Autodesk Inventor part; units mm, degrees
ref_plane "Work Plane1" through (-2, 0, -9) normal (-1, 0, 0) x (0, 0, 1)
ref_plane "Work Plane2" through (-2.4, 12.4824, -5.5) normal (0, 0, 1) x (1, 0, 0)
ref_plane "YZ Plane" through (0, 0, 0) normal (1, 0, 0) x (0, 1, 0)
sketch "Sketch1" plane through (0, 0, 0) normal (0, 1, 0) x (-1, 0, 0)
  line L0 (0, 0) -> (4, 0)
  line L1 (4, 0) -> (4, -11)
  line L2 (4, -11) -> (0, -11)
  line L3 (0, -11) -> (0, 0)
  dimension "d0" = 4
  dimension "d1" = 11
extrude "Extrusion1" add sketch "Sketch1" along normal blind 9.3
sketch "Sketch2" plane through (0, 9.3, 0) normal (0, 1, 0) x (1, 0, 0)
  line L0 (-4, 0) -> (0, 0)
  line L1 (0, 0) -> (0, 11)
  line L2 (0, 11) -> (-4, 11) construction
  line L3 (-4, 11) -> (-4, 0)
  line L4 (0, 11) -> (-4, 11) construction
  line L5 (-2.4, 0.15) -> (-1.6, 0.15)
  line L6 (-1.6, 0.15) -> (-1.6, 10.85)
  line L7 (-1.6, 10.85) -> (-2.4, 10.85)
  line L8 (-2.4, 10.85) -> (-2.4, 0.15)
  dimension "d5" = 0.8
  dimension "d6" = 4
  dimension "d7" = 1.6
  dimension "d40" = 0.15
  dimension "d41" = 0.15
extrude "Extrusion2" add sketch "Sketch2" along normal blind 7.3
sketch "Sketch3" plane through (-1.6, 9.3, -0.15) normal (1, 0, 0) x (0, 0, -1)
  line L0 (10.7, 0) -> (0, 0)
  line L1 (10.7, 0) -> (10.7, 7.3)
  line L2 (0, 7.3) -> (10.7, 7.3)
  line L3 (0, 0) -> (0, 7.3)
  line L4 (0, 7.3) -> (10.7, 7.3)
  line L5 (0, 0) -> (10.7, 0)
  line L6 (3, 7.3) -> (7.7, 7.3)
  line L7 (7.7, 7.3) -> (7.7, 0)
  line L8 (7.7, 0) -> (3, 0)
  line L9 (3, 0) -> (3, 7.3)
  point P0 (-0.15, -9.3)
  dimension "d10" = 3
  dimension "d11" = 3
extrude "Extrusion3" cut sketch "Sketch3" against normal blind 9.3 contours L0 L9 L2 L7
chamfer "Chamfer1" distance 0.85 distance2 3.5 1 edges at (-2, 16.6, -3.15) measured on face at (-2.1333, 16.6, -2.15)
chamfer "Chamfer2" distance 0.85 distance2 3.5 1 edges at (-2, 16.6, -0.15) measured on face at (-2.1333, 16.6, -1.5833)
chamfer "Chamfer3" distance 0.85 distance2 3.5 1 edges at (-2, 16.6, -7.85) measured on face at (-2.1333, 16.6, -9.85)
chamfer "Chamfer4" distance 0.85 distance2 3.5 1 edges at (-2, 16.6, -10.85) measured on face at (-2.1333, 16.6, -10.1333)
sketch "Sketch4" plane through (0, 0, 0) normal (0, -1, 0) x (1, 0, 0)
  line L0 (0, 0) -> (-4, 0)
  line L1 (-4, 0) -> (-4, -11)
  line L2 (-4, -11) -> (0, -11)
  line L3 (0, -11) -> (0, 0)
  line L4 (-2, -2) -> (-2, -9) construction
  line L5 (-4, -2) -> (-4, -9)
  line L6 (0, -9) -> (0, -2)
  arc A0 (0, -2) -> (-4, -2) centre (-2, -2) ccw
  arc A1 (-4, -9) -> (0, -9) centre (-2, -9) ccw
  line L7 (0, 0) -> (-4, 0)
  line L8 (0, -11) -> (0, 0)
  point P0 (-2, -5.5)
extrude "Extrusion4" cut sketch "Sketch4" against normal blind 0.5 contours L3 A0 L0 | A0 L1 L0 | L3 L2 A1 | A1 L2 L1
sketch "Sketch5" plane through (-4, 9.3, -11) normal (-1, 0, 0) x (0, 0, 1)
  line L0 (0, -8.8) -> (2, -8.8)
  line L1 (2, -8.8) -> (2, -9.3)
  line L2 (9, -9.3) -> (2, -9.3) construction
  line L3 (9, -8.8) -> (9, -9.3)
  line L4 (9, -8.8) -> (11, -8.8)
  line L5 (11, -8.8) -> (11, 0)
  line L6 (0, 0) -> (11, 0)
  line L7 (0, -8.8) -> (0, 0)
  line L8 (10.1, 0) -> (8.5, 0)
  line L9 (8.5, 0) -> (8.5, -7.8)
  line L10 (8.5, -7.8) -> (10.1, -7.8)
  line L11 (10.1, -7.8) -> (10.1, 0)
  line L12 (11, 0) -> (0, 0)
  line L13 (0.9, 0) -> (2.5, 0)
  line L14 (2.5, 0) -> (2.5, -7.8)
  line L15 (2.5, -7.8) -> (0.9, -7.8)
  line L16 (0.9, -7.8) -> (0.9, 0)
  point P0 (11, -9.3)
  dimension "d28" = 0.9
  dimension "d29" = 0.9
  dimension "d30" = 1.6
  dimension "d31" = 1.6
  dimension "d32" = 1.5
extrude "Extrusion5" cut sketch "Sketch5" against normal blind 0.8
ref_plane "Work Plane1" through (-2, 0, -9) normal (-1, 0, 0) x (0, 0, 1)
mirror "Mirror1" about plane through (-2, 0, -9) normal (-1, 0, 0) of "Extrusion5"
sketch "Sketch6" plane through (-1.6, 9.3, 0) normal (0, 0, 1) x (1, 0, 0)
  line L0 (0.8, 0) -> (0.8, -7.8)
  line L1 (0.8, -7.8) -> (0.8, 0)
  line L2 (-1.6, -7.8) -> (-1.6, 0)
  line L3 (0.8, 0) -> (0.8, -7.8)
  line L4 (0.8, -3.5) -> (1.6, -5.3)
  line L5 (1.6, 0) -> (1.6, -7.8)
  line L6 (-2.4, -9.3) -> (1.6, -9.3)
  line L7 (0.8, 0) -> (1.6, 0)
  line L8 (0.8, 0) -> (1.6, 0)
  dimension "d36" = 3.5
  dimension "d37" = 4
extrude "Extrusion6" cut sketch "Sketch6" against normal blind 1.2
mirror "Mirror2" about plane through (-2, 0, -9) normal (-1, 0, 0) of "Extrusion6"
ref_plane "Work Plane2" through (-2.4, 12.4824, -5.5) normal (0, 0, 1) x (1, 0, 0)
mirror "Mirror3" about plane through (-2.4, 12.4824, -5.5) normal (0, 0, 1) of "Extrusion6", "Mirror2"
equation "\"d7\" = -0.5 * d5 + 0.5 * d6"
equation "\"d31\" = d30"
properties part number "Mini car fuse"
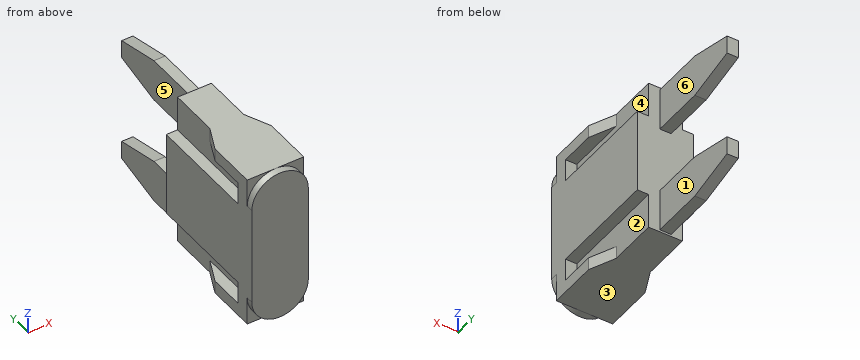
Could you check a few things on this model? Use its own coordinates, in mm. Face numbers are marked on the shaded views. A direction names the side the tool comes from. Give positions to 0.01 mm unless a question says otherwise; leave off trailing zeros. Loops run counter-clockwise (first coordinate to the right, second up) from the corner with the lowest first, then second, coordinate; pieces in that order, holes last. Notation, with made-up numbers: (-23.5, 40) -> (19.5, 40) arc R23 ccw to (19.5, 74) -> close; hole circle Ø9 at (52.25, 35). An arc over 180 degrees is marked (long way). Return JSON: item names as keys, results as strings.
Item 1: Which directions (+Z, -Z, +X, -X, +Y, -Y) give clear straight access to the entire face, cutting with the end or side of a thin tool? Please do the marked faces 4, 5 and 6.
Geometry results:
{"face 4": "+X, +Y", "face 5": "+Z, -Z, -X, +Y", "face 6": "+Z, -Z, +X, +Y"}
Item 2: I'm going to push flat-ended pins straight in: pin 1 (1 mm diameter, centred on y = 10, z = -4, fed in from -X); pin 2 (1.5 mm diameter, centred on y = 11.5, z = -1.5, fed in from -X); pin 3 (0.6 mm diameter, centred on x = 0, z = -9.5, fed in from +Y); pin 4 (1 mm diameter, centred on y = 2.5, z = -9.5, fed in from -X). Where does each tip first touch, or does it pass through?
Geometry results:
{"pin 1": "passes through", "pin 2": "stops at x = -2.4", "pin 3": "stops at y = 1.5", "pin 4": "stops at x = -3.2"}
Item 3: If we section it at D-D on z = -7: List the corners of the cut face in (x, y) for me, plus the area to 3 significant figures.
Geometry results:
{"outline": "(-4, 0) -> (0, 0) -> (0, 9.3) -> (-4, 9.3) -> close", "area": "37.2 mm²"}
Item 4: If we section it at A-A on y = 12.25: List the corners of the cut face in (x, z) for me, plus the area to 3 significant figures.
Geometry results:
{"outline": "(-2.4, -10.85) -> (-1.6, -10.85) -> (-1.6, -7.85) -> (-2.4, -7.85) -> close; (-2.4, -3.15) -> (-1.6, -3.15) -> (-1.6, -0.15) -> (-2.4, -0.15) -> close", "area": "4.80 mm²"}
Item 5: If we section it at C-C on y = 5.5: List the corners of the cut face in (x, z) for me.
Geometry results:
{"outline": "(-4, -8.5) -> (-3.2, -8.5) -> (-3.2, -10.1) -> (-3.33, -10.1) -> (-3.33, -11) -> (-0.67, -11) -> (-0.67, -10.1) -> (-0.8, -10.1) -> (-0.8, -8.5) -> (0, -8.5) -> (0, -2.5) -> (-0.8, -2.5) -> (-0.8, -0.9) -> (-0.67, -0.9) -> (-0.67, 0) -> (-3.33, 0) -> (-3.33, -0.9) -> (-3.2, -0.9) -> (-3.2, -2.5) -> (-4, -2.5) -> close"}
Item 6: We'd pull the mould along Z, two halves only. Please class the marked faces 1, 2 and 3: +Z half, -Z half, draft (parallel to the pull), parting line (faces both ways), or undercut.
Geometry results:
{"face 1": "draft", "face 2": "undercut", "face 3": "-Z half"}
Item 7: I need wall thicknesses on L1, parallel to Z at x = -3.7, y = 2.25; L2, parallel to Y at x = -0.8, z = -8.25; L3, parallel to X at y = 15.75, z = -1. Which ranges of each line are inside material? Lowest first, please. Write a range as from..to.
Geometry results:
{"L1": "z = -11..-10.1, -8.5..-2.5, -0.9..0", "L2": "y = 0..9.3", "L3": "x = -2.4..-1.6"}
Item 8: If we section it at B-B on x = -3.6: List the corners of the cut face in (y, z) for me.
Geometry results:
{"outline": "(0, -10.2) -> (0.5, -10.2) -> (0.5, -11) -> (4.9, -11) -> (4.9, -10.1) -> (1.5, -10.1) -> (1.5, -8.5) -> (9.3, -8.5) -> (9.3, -2.5) -> (1.5, -2.5) -> (1.5, -0.9) -> (4.9, -0.9) -> (4.9, 0) -> (0.5, 0) -> (0.5, -0.8) -> (0, -0.8) -> close"}
